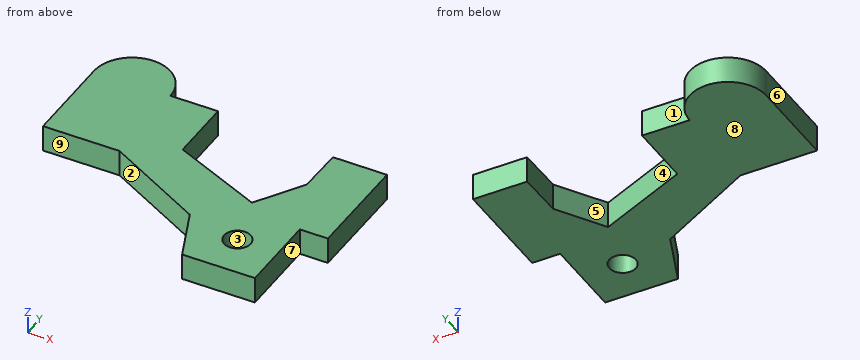
```python
from build123d import *

# Parameters (mm, degrees)
F0_R     = 2
F1_DEPTH = 4


with BuildPart() as f1:
    # F0 (on Top) → F1 (new body)
    with BuildSketch(Plane.XY):
        with BuildLine():
            Line((-159.543321, 56.417756), (-159.543321, 42.404792))
            Line((-159.543321, 42.404792), (-148.025898, 42.404792))
            Line((-148.025898, 42.404792), (-133.070684, 34.393251))
            Line((-133.070684, 34.393251), (-129.709324, 26.128011))
            Line((-129.709324, 26.128011), (-118.751742, 26.128011))
            Line((-118.751742, 26.128011), (-118.751742, 38.491473))
            Line((-118.751742, 38.491473), (-114.518747, 38.478882))
            Line((-114.518747, 38.478882), (-114.470554, 54.681407))
            Line((-114.470554, 54.681407), (-122.62332, 54.705656))
            Line((-122.62332, 54.705656), (-122.733846, 47.726375))
            Line((-122.733846, 47.726375), (-127.154761, 40.680661))
            Line((-127.154761, 40.680661), (-140.857846, 46.682025))
            Line((-140.857846, 46.682025), (-140.857846, 56.417756))
            Line((-140.857846, 56.417756), (-148.025898, 56.417756))
            ThreePointArc((-148.025898, 56.417756), (-153.784609, 62.176467), (-159.543321, 56.417756))
        make_face()
        with Locations((-124.899976, 32.55615)):
            Circle(F0_R, mode=Mode.SUBTRACT)
    extrude(amount=F1_DEPTH)


solid = f1.part
```
Geometry: final body of the model. Coordinates: model frame, mm. Face numbers are marked on the shaded views. A direction names the side the tool comes from. Round coordinates to 2 decimals unless told otherwise and drop trailing zeros. Order: outer loops, then holes, each group sorted by start corner. A loop starts at its lowest first (then second) coordinate and runs counter-clockwise, first axis right, second up. Notation, with made-up numbers: (80.25, 68) - (90.25, 68) arc R15 ccw to (90.25, 86) - close; hole circle Ø4 at (45.25, 18). An arc over 180 degrees is marked (long way). Write item = value, one per line. Start each with the question number.
Q1. Pull-direction query (X, two-part tool) for the marked faces 1, 2, 3 and 4; classes: +X half, -X half, draft (parallel to the pull), parting line (faces both ways), or undercut.
Q2. Pin query (flat end, axial travel): pin 1 (2 mm diameter, centred on x = -136, z = 0.5, fed in from +Y); pin 2 (5 mm diameter, centred on x = -141.5, y = 56.5, fed in from -Z); pin 3 (2 mm diameter, centred on x = -155, z = 1.5, fed in from -Y). Return the tip coordinate at first contact, or that it passes through.
Q3. Cut plane D-D on x = -154. Return the cut outline in (y, z), and give its area (3 significant figures).
Q4. Cut plane C-C on z = 2.7. Return the cut outline in (x, y), and give its area (3 significant figures).
Q5. Ray query, line 1 (X direction, y = 46, z = 1.8); line 2 (X direction, y = 56.5, z = 2.2); line 3 (X direction, y = 45, z = 1.85). Return the intervals inside material, ascending. Write a range as from..to.
Q6. Cut plane A-A on y = 41.5. Return the cut outline in (x, z).
Q7. Access query for the marked faces 5, 6, 7, 8 and 9. Directions: +Z, -Z, +X, -X, +Y, -Y. A direction counts if a zero-diameter tool reaches every point of the face in a straight line with its end or side. Return the directions, or none.
Q8. Cut plane B-B on x = -124.5. Return the cut outline in (y, z), and give its area (3 significant figures).
Outcome:
q1.face_1 = draft
q1.face_2 = -X half
q1.face_3 = undercut
q1.face_4 = undercut
q2.pin_1 = 44.99
q2.pin_2 = 0
q2.pin_3 = 42.4
q3.outline = (42.4, 0) - (62.17, 0) - (62.17, 4) - (42.4, 4) - close
q3.area = 79.1 mm^2
q4.outline = (-159.54, 42.4) - (-148.03, 42.4) - (-133.07, 34.39) - (-129.71, 26.13) - (-118.75, 26.13) - (-118.75, 38.49) - (-114.52, 38.48) - (-114.47, 54.68) - (-122.62, 54.71) - (-122.73, 47.73) - (-127.15, 40.68) - (-140.86, 46.68) - (-140.86, 56.42) - (-148.03, 56.42) arc R5.76 ccw to (-159.54, 56.42) - close; hole circle Ø4 at (-124.9, 32.56)
q4.area = 723 mm^2
q5.line_1 = -159.54..-139.3, -123.82..-114.5
q5.line_2 = -159.54..-148.03
q5.line_3 = -159.54..-137.02, -124.44..-114.5
q6.outline = (-146.34, 0) - (-129.03, 0) - (-129.03, 4) - (-146.34, 4) - close; (-126.64, 0) - (-114.51, 0) - (-114.51, 4) - (-126.64, 4) - close
q7.face_5 = +Z, -Z, +Y
q7.face_6 = +Z, -Z, -X, +Y, -Y
q7.face_7 = +Z, -Z, +X, -Y
q7.face_8 = -Z, +X, -X, +Y, -Y
q7.face_9 = +Z, -Z, -X, -Y
q8.outline = (26.13, 0) - (30.6, 0) - (30.6, 4) - (26.13, 4) - close; (34.52, 0) - (44.91, 0) - (44.91, 4) - (34.52, 4) - close
q8.area = 59.5 mm^2
